```python
from build123d import *

# Parameters (mm, degrees)
SKETCH1_W           = 60
SKETCH1_H           = 6
BASE_DEPTH          = 2
BOSS_EXTRUDE2_DEPTH = 6
FILLET1_R           = 2
CROP_REACH          = 33.193
FAN_SCREWS_REACH    = 33.623
SKETCH5_R           = 1.4
PCB_SCREWS_REACH    = 33.193
SKETCH3_R           = 1.4


with BuildPart() as part:
    # Sketch1 → Base (new body)
    with BuildSketch(Plane.XY):
        Rectangle(SKETCH1_W, SKETCH1_H)
    extrude(amount=BASE_DEPTH)

    # Sketch4 → Boss-Extrude2 (add)
    with BuildSketch(Plane(origin=(0, -3, 0), x_dir=(1, 0, 0), z_dir=(0, 1, 0))):
        Polygon((-30, -2), (-18, -2), (-18, -8), (-25, -8), (-30, -8), align=None)
        Polygon((30, -2), (30, -8), (25, -8), (18, -8), (18, -2), align=None)
    extrude(amount=BOSS_EXTRUDE2_DEPTH)

    # Fillet1
    fillet1_edges = [part.edges().sort_by_distance(p)[0] for p in [
        (-18, 0, 2),
        (-18, 0, 8),
        (-30, 0, 8),
        (30, 0, 8),
        (18, 0, 8),
        (18, 0, 2),
    ]]
    fillet(fillet1_edges, radius=FILLET1_R)

    # Sketch2 → Crop (cut, up to next)
    with BuildSketch(Plane.XY, mode=Mode.PRIVATE) as crop_sk1:
        Polygon((-25.875432474, 3), (-29.339534089, -3), (-30, -3), (-30, 3), align=None)
    crop_tool1 = extrude(crop_sk1.sketch, amount=CROP_REACH, mode=Mode.PRIVATE) & part.part
    add(crop_tool1.solids().sort_by_distance((-28.594757, 0.723945, 0))[0], mode=Mode.SUBTRACT)

    # Sketch5 → Fan screws (cut, up to next)
    with BuildSketch(Plane.XZ.offset(3), mode=Mode.PRIVATE) as fan_screws_sk1:
        with Locations(Location((25, 5, 0), (0, 0, 270))):
            Circle(SKETCH5_R)
    fan_screws_tool1 = extrude(fan_screws_sk1.sketch, amount=-FAN_SCREWS_REACH, mode=Mode.PRIVATE) & part.part
    # Sketch5 → Fan screws (cut, up to next)
    with BuildSketch(Plane.XZ.offset(3), mode=Mode.PRIVATE) as fan_screws_sk2:
        with Locations(Location((-25, 5, 0), (0, 0, 270))):
            Circle(SKETCH5_R)
    fan_screws_tool2 = extrude(fan_screws_sk2.sketch, amount=-FAN_SCREWS_REACH, mode=Mode.PRIVATE) & part.part
    add(fan_screws_tool1.solids().sort_by_distance((25, -3, 5))[0], mode=Mode.SUBTRACT)
    add(fan_screws_tool2.solids().sort_by_distance((-25, -3, 5))[0], mode=Mode.SUBTRACT)

    # Sketch3 → PCB screws (cut, up to next)
    with BuildSketch(Plane.XY, mode=Mode.PRIVATE) as pcb_screws_sk1:
        with Locations(Location((21.448, -0.1262, 0), (0, 0, 180))):
            Circle(SKETCH3_R)
    pcb_screws_tool1 = extrude(pcb_screws_sk1.sketch, amount=PCB_SCREWS_REACH, mode=Mode.PRIVATE) & part.part
    # Sketch3 → PCB screws (cut, up to next)
    with BuildSketch(Plane.XY, mode=Mode.PRIVATE) as pcb_screws_sk2:
        with Locations(Location((-21.552, -0.1262, 0), (0, 0, 180))):
            Circle(SKETCH3_R)
    pcb_screws_tool2 = extrude(pcb_screws_sk2.sketch, amount=PCB_SCREWS_REACH, mode=Mode.PRIVATE) & part.part
    add(pcb_screws_tool1.solids().sort_by_distance((21.448, -0.1262, 0))[0], mode=Mode.SUBTRACT)
    add(pcb_screws_tool2.solids().sort_by_distance((-21.552, -0.1262, 0))[0], mode=Mode.SUBTRACT)


solid = part.part
```
CAD build for the part. Positions are in the model's coordinates, mm. A direction names the side the tool comes from. Round coordinates to 2 decimals unless told otherwise and drop trailing zeros. Write each loop counter-clockwise with the first axis right and the second up, starting at its lowest first coordinate (ties: lowest second). Pieces come first, ordered by that corner, then holes. Notation, with made-up numbers: (55, 14.5) -> (65, 14.5) arc R32 ccw to (65, 43.5) -> close; hole circle Ø9 at (89.25, -21.5). An arc over 180 degrees is marked (long way). Answer in a Markdown table with one row per item. Add a question column.
Item 1: Drill centre lines: line 1 (X direction, y = 2.5, z = 5.25); line 2 (Z direction, x = -25, y = 2.25); line 3 (X direction, y = -0.25, z = 5). Where is each one in solid material? Low to high. Write a range as from..to.
Item 2: Saw through at C-C, the plane z = 2.75. Write the cut outline in (x, y), then the cut area to 3 significant figures.
Item 3: Saw through at B-B, the plane y = 0.5. Write the cut outline in (x, z), then the cut area to 3 significant figures.
Item 4: Saw through at D-D, the plane z = 5. Write the cut outline in (x, y), then the cut area to 3 significant figures.
Item 5: Which spindle directions (+Z, -Z, +X, -X, +Y, -Y) get a long thin tool onto all of the face, cutting with end or side? Do faces 1 (the face through (-24, 0, 8)), 2 (the face through (-17.43, 0.04, 2.6)). Say none if no direction does.
Item 6: Mould opens along X. For faces 3 (the face through (30, 0, 3)), 4 (the face through (-18, 0, 5)), 5 (the face through (-27.583, 0.042, 3.944)), 6 (the face through (0, 0, 0)) say: pulls with the +X half, pulls with the -X half, needs draft (parallel to the pull), parting line crosses it, or undercut.
Item 7: Drop flat-ended pins along their axis: pin 1 Ø3 at (x, y) = (11.5, -1.5) entering from -Z; pin 2 Ø2 at (y, z) = (1, 4.5) entering from -X; pin 3 Ø1.5 at (y, z) = (-1.5, 3.5) entering from -X; pin 4 Ø1.5 at (y, z) = (1, 5) entering from -X. Give the stop position or say it passes through.
Item 8: Saw through at A-A, the plane x = -25. Write the cut outline in (y, z).
Findings below:
| question | item | result |
|---|---|---|
| 1 | line 1 | x = -23.62..-18, 18..23.62, 26.38..30 |
| 1 | line 2 | z = 0..3.6, 6.4..8 |
| 1 | line 3 | x = -27.75..-26.4, -23.6..-22.95, -20.16..-18, 18..20.05, 22.84..23.6, 26.4..30 |
| 2 | outline | (-29.34, -3) -> (-17.56, -3) -> (-17.56, 3) -> (-25.88, 3) -> close; (17.56, -3) -> (30, -3) -> (30, 3) -> (17.56, 3) -> close; hole circle Ø2.8 at (-21.55, -0.13); hole circle Ø2.8 at (21.45, -0.13) |
| 2 | area | 123 mm^2 |
| 3 | outline | (-27.32, 0) -> (-22.8, 0) -> (-22.8, 8) -> (-27.32, 8) -> close; (-20.3, 0) -> (20.2, 0) -> (20.2, 8) -> (20, 8) arc R2 ccw to (18, 6) -> (18, 4) arc R2 cw to (16, 2) -> (-16, 2) arc R2 cw to (-18, 4) -> (-18, 6) arc R2 ccw to (-20, 8) -> (-20.3, 8) -> close; (22.7, 0) -> (30, 0) -> (30, 6) arc R2 ccw to (28, 8) -> (22.7, 8) -> close; hole circle Ø2.8 at (-25, 5); hole circle Ø2.8 at (25, 5) |
| 3 | area | 189 mm^2 |
| 4 | outline | (-29.34, -3) -> (-26.4, -3) -> (-26.4, 2.09) -> close; (-23.6, -3) -> (-18, -3) -> (-18, 3) -> (-23.6, 3) -> close; (18, -3) -> (23.6, -3) -> (23.6, 3) -> (18, 3) -> close; (26.4, -3) -> (30, -3) -> (30, 3) -> (26.4, 3) -> close; hole circle Ø2.8 at (-21.55, -0.13); hole circle Ø2.8 at (21.45, -0.13) |
| 4 | area | 84.0 mm^2 |
| 5 | face 1 | +Z, +X, -X, +Y, -Y |
| 5 | face 2 | +Z, +Y, -Y |
| 6 | face 3 | pulls with the +X half |
| 6 | face 4 | undercut |
| 6 | face 5 | pulls with the -X half |
| 6 | face 6 | needs draft |
| 7 | pin 1 | stops at z = 0 |
| 7 | pin 2 | stops at x = -27.61 |
| 7 | pin 3 | stops at x = -28.91 |
| 7 | pin 4 | stops at x = -27.46 |
| 8 | outline | (-3, 0) -> (3, 0) -> (3, 3.6) -> (-3, 3.6) -> close; (-3, 6.4) -> (3, 6.4) -> (3, 8) -> (-3, 8) -> close |
